Source: CAD feature listing. Evaluate the final solid. Frame: model axes, mm. Face numbers are marked on the shaded views. A direction names the side the tool comes from. Give positions to 0.01 mm unless a question says otherwise; leave off trailing zeros. Order: outer loops, then holes, each group sorted by start corner. A loop starts at its lowest first (then second) coordinate and runs counter-clockwise, first axis right, second up. Notation, with made-up numbers: M 45,52 L 76,52 A21 ccw 76,75 Z; hole C 25.25,-39.75 d10. An arc over 180 degrees is marked long. Answer as a JSON object with one key per item and string values. Group by question number.
1. Pin query (flat end, axial travel): P1, Ø10, axis at y = -31.5, z = 16.5, coming from the -X side; P2, Ø1.5, axis at x = 20, z = -22.5, coming from the +Y side; P3, Ø20, axis at x = -17, y = -65, coming from the -Z side; P4, Ø1.4, axis at x = 25, z = -2.5, coming from the -Y side. Return the tip coordinate at first contact, or that it passes through.
2. Section query D-D (y = -50). Output: boundary loops of the cut face in (x, z), plus the area to 3 significant figures.
3. Section query B-B (y = -13.5). Output: boundary loops of the cut face in (x, z).
4. Pull-direction query (Y, two-part tool) for the marked faces 4, 5, 6 and 7; classes: +Y half, -Y half, draft (parallel to the pull), parting line (faces both ways), or undercut.
5. Set-up query: the marked faces 1, 2 and 3. Return all of +Z, -Z, +X, -X, +Y, -Y with unobstructed straight access to the full face (end or side cutting, diameter ignored); none if empty.
6. Section query C-C (y = -70.5). Output: boundary loops of the cut face in (x, z), plus the area to 3 significant figures.
7. Section query A-A (z = 0). Output: boundary loops of the cut face in (x, y).
8. Material intervals for L1, parallel to Y at x = -23, z = 8.5; L2, parallel to Y at x = -19, z = -18; L3, parallel to Y at x = -13, z = -10.5, sorted ascending. Write a range as [from, to].
from build123d import *

# Parameters (mm, degrees)
F0_R     = 36.052537
F1_DEPTH = 42.5522
F2_R     = 10.384305
F4_DEPTH = 12.7


with BuildPart() as f1:
    # F0 (on Front) → F1 (new body)
    with BuildSketch(Plane.XZ):
        Circle(F0_R)
    extrude(amount=F1_DEPTH)

    # F2
    f2_edges = [f1.edges().sort_by_distance(p)[0] for p in [
        (-36.052537, -42.5522, 0),
    ]]
    fillet(f2_edges, radius=F2_R)

    # F3 (on Top) → F4 (join, symmetric)
    with BuildSketch(Plane.XY):
        Polygon((24.906132, -41.96053), (-25.40835, -43.80627), (-18.461386, -55.194348), (-31.700424, -63.270436), (17.599434, -82.260892), (20.955874, -73.547461), (4.182442, -67.086284), (23.552079, -57.608064), (0, -57.608064), align=None)
    extrude(amount=F4_DEPTH, both=True)


solid = f1.part
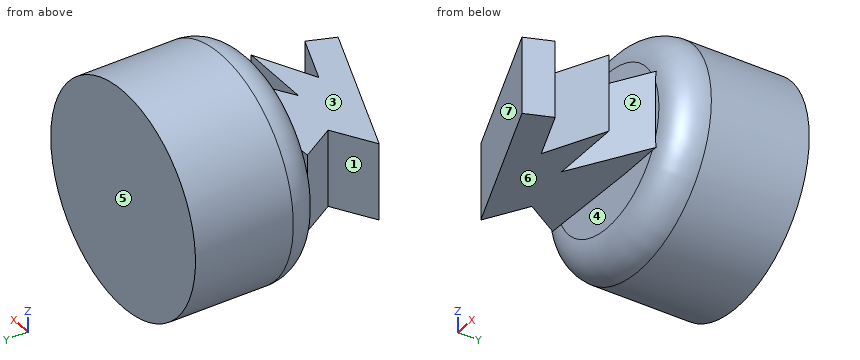
Answer sheet:
{
 "1": {"P1": "x = -34.17", "P2": "y = 0", "P3": "z = -12.7", "P4": "y = -42.55"},
 "2": {"outline": "M -21.63,-12.7 L 12.11,-12.7 L 12.11,12.7 L -21.63,12.7 Z", "area": "857 mm^2"},
 "3": {"outline": "C 0,0 d72.11"},
 "4": {"face 4": "undercut", "face 5": "+Y half", "face 6": "draft", "face 7": "-Y half"},
 "5": {"face 1": "+Z, -Z, -X", "face 2": "+Z, -Z, +X", "face 3": "+Z, +X, -X, -Y"},
 "6": {"outline": "M -12.93,-12.7 L 13.04,-12.7 L 13.04,12.7 L -12.93,12.7 Z", "area": "660 mm^2"},
 "7": {"outline": "M -36.05,-32.17 A10.38 ccw -25.67,-42.55 L 8.78,-42.55 L -25.41,-43.81 L -18.46,-55.19 L -31.7,-63.27 L 17.6,-82.26 L 20.96,-73.55 L 4.18,-67.09 L 23.55,-57.61 L 0,-57.61 L 23.96,-42.55 L 25.67,-42.55 A10.38 ccw 36.05,-32.17 L 36.05,0 L -36.05,0 Z"},
 "8": {"L1": "[-66.62, -57.96], [-47.75, -43.72], [-42.55, 0]", "L2": "[-42.54, 0]", "L3": "[-70.47, -43.35], [-42.55, 0]"}
}
